Here's the drawing with two shaded views (mm, measured from the low corner). I have some questions. A direction names the side the tool comes from. Round coordinates to 2 decimals unless told otherwise and drop trailing zeros. Loops run counter-clockwise (first coordinate to the right, second up) from the corner with the lowest first, then second, coordinate; pieces in that order, holes last. Notation, with made-up numbers: (37, 71) - (49, 71) arc R29 cw to (49, 97) - close; hole circle Ø2 at (-9.75, 7.25). An arc over 180 degrees is marked (long way). Answer as CSV lines item,"result".
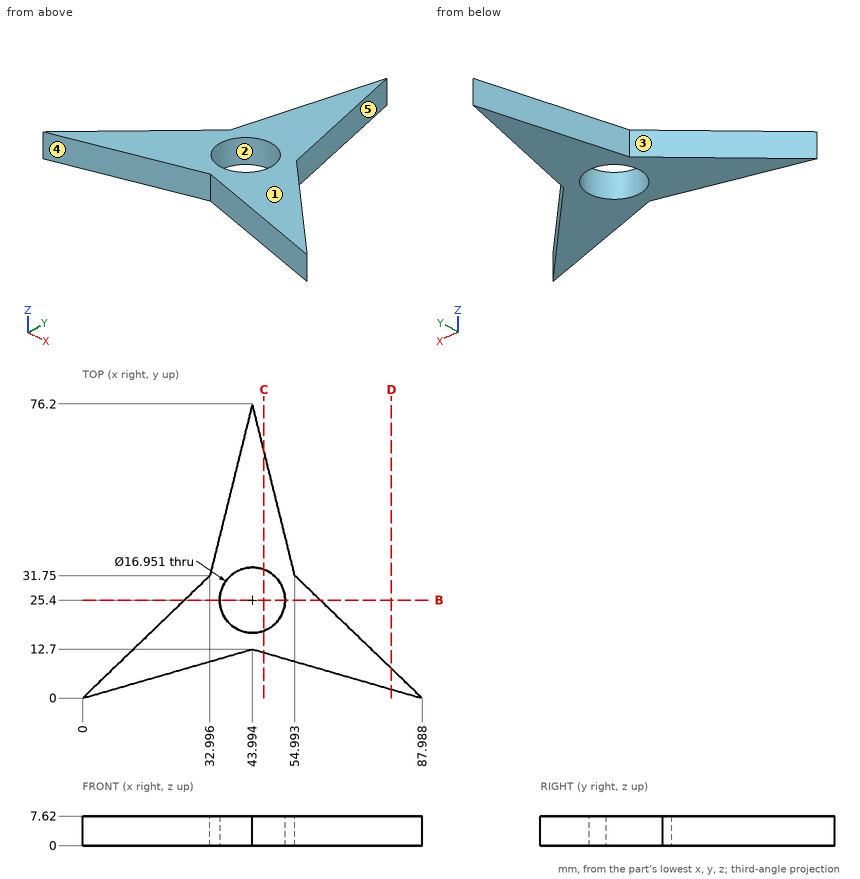
Q1. I'm going to push a flat-ended pin straight in: pin 1 Ø2 at (y, z) = (16, 2.5) entering from +X. Where does the tip first touch, or does it pass through?
Checks:
pin 1,"x = 72.4"
Q2. If I drill on line 1 along X through (y, z) = (25.4, 6) (1 decimal); line 2 along Y through (x, z) = (79.5, 6.75); line 3 along Y through (x, z) = (16, 3.5) (1 decimal), over which ranges is the centre line in solid material (lowest first)? Write a range as [from, to].
Checks:
line 1,"[26.4, 35.5], [52.5, 61.6]"
line 2,"[2.45, 8.17]"
line 3,"[4.6, 15.4]"
Q3. Imagine slicing it at D-D (x = 80). Write out the boundary of the cut face in (y, z).
Checks:
outline,"(2.31, 0) - (7.69, 0) - (7.69, 7.62) - (2.31, 7.62) - close"
Q4. On a 3-axis mill with a long thin cutter (end or side, diameter ignored), from which of +Z, -Z, +X, -X, +Y, -Y can I reach the whole of each face in a straight line? I mean the marked faces 4 and 5. Say none if no direction works.
Checks:
face 4,"+Z, -Z, -Y"
face 5,"+Z, -Z, +X, +Y"
Q5. We'd pull the mould along X, two halves only. Please class the marked faces 1, 2 and 3: pulls with the +X half, pulls with the -X half, needs draft (parallel to the pull), parting line crosses it, or undercut.
Checks:
face 1,"needs draft"
face 2,"undercut"
face 3,"pulls with the -X half"
Q6. Imagine slicing it at B-B (y = 25.4). Write out the boundary of the cut face in (x, z).
Checks:
outline,"(26.4, 0) - (35.52, 0) - (35.52, 7.62) - (26.4, 7.62) - close; (52.47, 0) - (61.59, 0) - (61.59, 7.62) - (52.47, 7.62) - close"
Q7. Imagine slicing it at C-C (x = 47). Write out the boundary of the cut face in (y, z) (1 decimal).
Checks:
outline,"(11.8, 0) - (17.5, 0) - (17.5, 7.6) - (11.8, 7.6) - close; (33.3, 0) - (64.1, 0) - (64.1, 7.6) - (33.3, 7.6) - close"
